Check sheet for the modelled part. Datum: model origin and axes. Units: mm. Round coordinates to 2 decimals unless told otherwise and drop trailing zeros. Loops run counter-clockwise (first coordinate to the right, second up) from the corner with the lowest first, then second, coordinate; pieces in that order, holes last. Notation, with made-up numbers: (-2, 32) -> (53, 32) arc R23 ccw to (53, 52) -> close; hole circle Ø3 at (-3, -1). An arc over 180 degrees is marked (long way). Use one line per item in the form item = value. Start each with the question number.
(1) Sectioned sample at C-C (z = -400). Record the cut outline in (x, y), and give its area (3 significant figures).
(2) Draft check along X on faces 1 (the flat face through (-750, 50, 7)), 2 (the flat face through (-10, 100, 254)), 3 (the cylindrical face through (589.575, 49.3, 393.491)), 4 (the cylindrical face through (589.575, 49.3, -406.509)). Enter one of: released by +X, released by -X, zero draft, split by the parting line, or undercut.
(3) Sectioned sample at B-B (y = 29). State how many separate pieces and enclosed holes the cut face has, and give its area (3 significant figures).
(4) Sectioned sample at D-D (x = 565.5). Record the cut outline in (y, z), and give its area (3 significant figures).
(5) Material ranges on probe 1 along X at (y, z) = (78.5, -400); probe 2 along Z at (x, y) = (-271.5, 87); probe 3 along Z at (x, y) = (300, 20), recorded low to high. Write a range as [from, to].
(6) Go/stop test with flat-tipped pins: pin 1 (0.8 mm diameter, centred on x = 208, y = 100.5, fed in from +Z); pin 2 (1.5 mm diameter, centred on x = 457.5, z = 213, fed in from +Y). Record where each tip stops, or that it passes through.
(7) Sectioned sample at A-A (x = -540). Record the cut outline in (y, z), and give its area (3 significant figures).
from build123d import *

# Parameters (mm, degrees)
SKETCH1_W           = 1500
SKETCH1_H           = 1000
SKETCH1_R           = 50
BOSS_EXTRUDE1_DEPTH = 100
BOSS_EXTRUDE2_DEPTH = 1


with BuildPart() as part:
    # Sketch1 → Boss-Extrude1 (new body)
    with BuildSketch(Plane(origin=(0, 0, 0), x_dir=(1, 0, 0), z_dir=(0, 1, 0))):
        Rectangle(SKETCH1_W, SKETCH1_H)
        with Locations(Location((-540, -400, 0), (0, 0, 270))):
            Circle(SKETCH1_R, mode=Mode.SUBTRACT)
        with Locations(Location((-270, -400, 0), (0, 0, 270))):
            Circle(SKETCH1_R, mode=Mode.SUBTRACT)
        with Locations(Location((0, -400, 0), (0, 0, 270))):
            Circle(SKETCH1_R, mode=Mode.SUBTRACT)
        with Locations(Location((270, -400, 0), (0, 0, 270))):
            Circle(SKETCH1_R, mode=Mode.SUBTRACT)
        with Locations(Location((540, -400, 0), (0, 0, 270))):
            Circle(SKETCH1_R, mode=Mode.SUBTRACT)
        with Locations(Location((-270, 400, 0), (0, 0, 270))):
            Circle(SKETCH1_R, mode=Mode.SUBTRACT)
        with Locations(Location((0, 400, 0), (0, 0, 270))):
            Circle(SKETCH1_R, mode=Mode.SUBTRACT)
        with Locations(Location((270, 400, 0), (0, 0, 270))):
            Circle(SKETCH1_R, mode=Mode.SUBTRACT)
        with Locations(Location((540, 400, 0), (0, 0, 270))):
            Circle(SKETCH1_R, mode=Mode.SUBTRACT)
        with Locations(Location((-540, 400, 0), (0, 0, 270))):
            Circle(SKETCH1_R, mode=Mode.SUBTRACT)
    extrude(amount=BOSS_EXTRUDE1_DEPTH)

    # Sketch2 → Boss-Extrude2 (add)
    with BuildSketch(Plane(origin=(0, 100, 0), x_dir=(1, 0, 0), z_dir=(0, 1, 0))):
        Polygon((-750, 0), (-750, 15), (750, 15), (750, -15), (-750, -15), align=None)
    extrude(amount=BOSS_EXTRUDE2_DEPTH)


solid = part.part
Checks:
q1.outline = (-750, 0) -> (-590, 0) -> (-590, 100) -> (-750, 100) -> close; (-490, 0) -> (-320, 0) -> (-320, 100) -> (-490, 100) -> close; (-220, 0) -> (-50, 0) -> (-50, 100) -> (-220, 100) -> close; (50, 0) -> (220, 0) -> (220, 100) -> (50, 100) -> close; (320, 0) -> (490, 0) -> (490, 100) -> (320, 100) -> close; (590, 0) -> (750, 0) -> (750, 100) -> (590, 100) -> close
q1.area = 100,000 mm2
q2.face_1 = released by -X
q2.face_2 = zero draft
q2.face_3 = undercut
q2.face_4 = undercut
q3.separate_pieces = 1
q3.enclosed_holes = 10
q3.area = 1,420,000 mm2
q4.outline = (0, -500) -> (100, -500) -> (100, -443.01) -> (0, -443.01) -> close; (0, -356.99) -> (100, -356.99) -> (100, -15) -> (101, -15) -> (101, 15) -> (100, 15) -> (100, 356.99) -> (0, 356.99) -> close; (0, 443.01) -> (100, 443.01) -> (100, 500) -> (0, 500) -> close
q4.area = 82,800 mm2
q5.probe_1 = [-750, -590], [-490, -320], [-220, -50], [50, 220], [320, 490], [590, 750]
q5.probe_2 = [-500, -449.98], [-350.02, 350.02], [449.98, 500]
q5.probe_3 = [-500, -440], [-360, 360], [440, 500]
q6.pin_1 = 15
q6.pin_2 = 100
q7.outline = (0, -500) -> (100, -500) -> (100, -450) -> (0, -450) -> close; (0, -350) -> (100, -350) -> (100, -15) -> (101, -15) -> (101, 15) -> (100, 15) -> (100, 350) -> (0, 350) -> close; (0, 450) -> (100, 450) -> (100, 500) -> (0, 500) -> close
q7.area = 80,000 mm2
